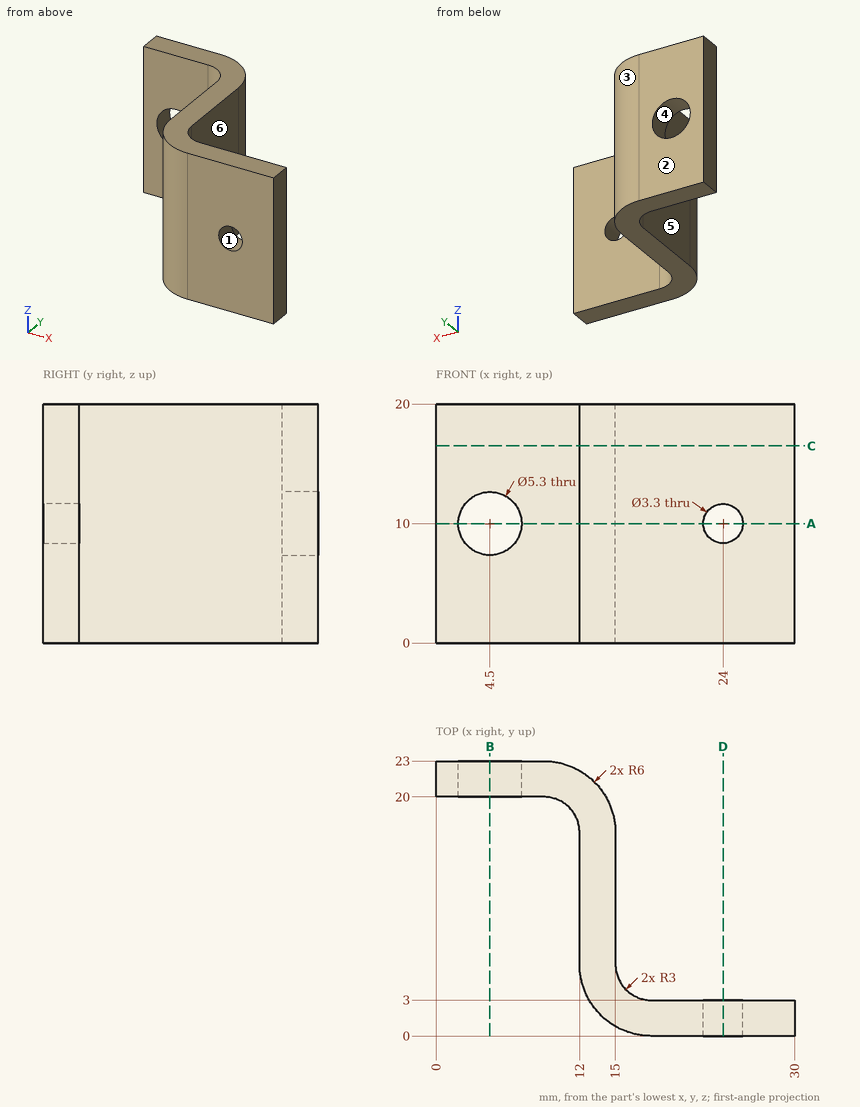
Verification items for this drawing (mm, ordinates from the low corner). A direction names the side the tool comes from. Give positions to 0.01 mm unless a question says otherwise; leave off trailing zeros. Loops run counter-clockwise (first coordinate to the right, second up) from the corner with the lowest first, then second, coordinate; pieces in that order, holes last. Notation, with made-up numbers: M 45,36 L 56,36 A13 cw 56,41 Z; hole C 4.25,2.25 d2. An arc over 180 degrees is marked long. Answer as a JSON object with one key per item and string values. Group by question number.
Q1. Go/stop test with flat-tipped pins: P1, Ø3, axis at y = 7.5, z = 9, coming from the -X side; P2, Ø2, axis at x = 8, z = 16.5, coming from the -Y side; P3, Ø4, axis at y = 16.5, z = 3.5, coming from the +X side. Record where each tip stops, or that it passes through.
Q2. Material ranges on line 1 along Y through (x, z) = (25.75, 3); line 2 along X through (y, z) = (7.25, 11.5); line 3 along X through (y, z) = (22.35, 10), recorded low to high. Write a range as [from, to].
Q3. Cross-section at B-B on x = 4.5. Record the cut outline in (y, z), then the cut area to 3 significant figures.
Q4. Release check for a two-part mould opening along X. For the marked faces 1, 2 and 3 record: released by +X, released by -X, zero draft, split by the parting line, or undercut.
Q5. Access from +Z, -Z, +X, -X, +Y, -Y to the whole of each face (thin tool, end or side, straight path). Record for the marked faces 4, 5 and 6.
Q6. Cross-section at C-C on z = 16.5. Record the cut outline in (x, y), then the cut area to 3 significant figures.
Q7. Cross-section at D-D on x = 24. Record the cut outline in (y, z), then the cut area to 3 significant figures.
Q8. Cross-section at A-A on z = 10. Record the cut outline in (x, y).
Evaluation:
{
 "1": {"P1": "stops at x = 12", "P2": "stops at y = 20", "P3": "stops at x = 15"},
 "2": {"line 1": "y = [0, 3]", "line 2": "x = [12, 15]", "line 3": "x = [0, 1.85], [7.15, 11.72]"},
 "3": {"outline": "M 20,0 L 23,0 L 23,7.35 L 20,7.35 Z; M 20,12.65 L 23,12.65 L 23,20 L 20,20 Z", "area": "44.1 mm2"},
 "4": {"face 1": "undercut", "face 2": "zero draft", "face 3": "released by +X"},
 "5": {"face 4": "+Y, -Y", "face 5": "+Z, -Z, -X, -Y", "face 6": "+Z, -Z, +X, +Y"},
 "6": {"outline": "M 0,20 L 9,20 A3 cw 12,17 L 12,6 A6 ccw 18,0 L 30,0 L 30,3 L 18,3 A3 cw 15,6 L 15,17 A6 ccw 9,23 L 0,23 Z", "area": "138 mm2"},
 "7": {"outline": "M 0,0 L 3,0 L 3,8.35 L 0,8.35 Z; M 0,11.65 L 3,11.65 L 3,20 L 0,20 Z", "area": "50.1 mm2"},
 "8": {"outline": "M 0,20 L 1.85,20 L 1.85,23 L 0,23 Z; M 7.15,20 L 9,20 A3 cw 12,17 L 12,6 A6 ccw 18,0 L 22.35,0 L 22.35,3 L 18,3 A3 cw 15,6 L 15,17 A6 ccw 9,23 L 7.15,23 Z; M 25.65,0 L 30,0 L 30,3 L 25.65,3 Z"}
}
